```python
from build123d import *

# Parameters (mm, degrees)
SKETCH1_W             = 92
SKETCH1_H             = 92
SKETCH1_R             = 0.51
BOSS_EXTRUDE1_DEPTH   = 1.59
CHAMFER1_SIZE         = 8.5
F_1_0MM_DOWEL_HOLE1_D = 3.18


with BuildPart() as part:
    # Sketch1 → Boss-Extrude1 (new body)
    with BuildSketch(Plane(origin=(0, 0, 0), x_dir=(1, 0, 0), z_dir=(0, 1, 0))):
        Rectangle(SKETCH1_W, SKETCH1_H)
        with Locations(Location((-2.67, -21.93, 0), (0, 0, 270))):
            Circle(SKETCH1_R, mode=Mode.SUBTRACT)
        with Locations(Location((2.03, -22.76, 0), (0, 0, 270))):
            Circle(SKETCH1_R, mode=Mode.SUBTRACT)
        with Locations(Location((-2.67, -42.06, 0), (0, 0, 270))):
            Circle(SKETCH1_R, mode=Mode.SUBTRACT)
        with Locations(Location((2.03, -41.24, 0), (0, 0, 270))):
            Circle(SKETCH1_R, mode=Mode.SUBTRACT)
    extrude(amount=BOSS_EXTRUDE1_DEPTH)

    # Chamfer1
    chamfer1_edges = [part.edges().sort_by_distance(p)[0] for p in [
        (46, 0.795, 46),
        (-46, 0.795, 46),
        (-46, 0.795, -46),
        (46, 0.795, -46),
    ]]
    chamfer(chamfer1_edges, length=CHAMFER1_SIZE)

    # Ø1.0mm Dowel Hole1 (through all)
    with Locations(Plane(origin=(0, 1.59, 0), x_dir=(1, 0, 0), z_dir=(0, 1, 0))):
        with Locations((-36.820611538, -35.589152958), (36.943757396, -37.559486686), (36.943757396, 39.283528698), (-36.820611538, 39.283528698)):
            Hole(F_1_0MM_DOWEL_HOLE1_D / 2)


solid = part.part
```
CAD build for the part. Positions are in the model's coordinates, mm. Round coordinates to 2 decimals unless told otherwise and drop trailing zeros. Return JSON: item names as keys, results as strings. Group by question number.
Q1. Two-plate mould, pull along X, no slides. Class faces 1 (the face through (38.116, 0.784, -40.358)), 2 (the face through (41.8, 0.8, 41.7)), 3 (the face through (-38.337, 0.784, 35.112)), 4 (the face through (-1, 1.59, -1)): +X half, -X half, draft (parallel to the pull), parting line (faces both ways), or undercut.
Q2. Drill centre lines: line 1 along X through (y, z) = (0.5, 22.76); line 2 along X through (y, z) = (0.25, 22). Where is each one in solid material? Low to high. Write a range as [from, to].
Q3. Band-saw the part on A-A on y = 0.85. Give the number of separate pieces and of enclosed holes in the cut face, plus the area to 3 significant figures.
Solutions:
{
 "1": {"face 1": "undercut", "face 2": "+X half", "face 3": "undercut", "face 4": "draft"},
 "2": {"line 1": "x = [-46, 1.52], [2.54, 46]", "line 2": "x = [-46, -3.18], [-2.16, 46]"},
 "3": {"separate pieces": "1", "enclosed holes": "8", "area": "8,280 mm^2"}
}
